Design review of the part shown in the three views and the two pictorial views. Dimensions are in mm from the part's minimum x, y and z. A direction names the side the tool comes from. Coordinates: 2 decimals unless noted, no trailing zeros. Write each loop counter-clockwise with the first axis right and the second up, starting at its lowest first coordinate (ties: lowest second). Pieces come first, ordered by that corner, then holes.
Q1. For pin 1 Ø5 at (x, y) = (6.5, 16.5) entering from +Z; pin 2 Ø2 at (x, y) = (15, 5) entering from +Z; pin 3 Ø1.8 at (x, y) = (9.5, 9) entering from +Z; pin 4 Ø2 at (x, z) = (4, 2) entering from -Y, all flat-tipped, find the tip position at first contact; note any pin that passes through.
Q2. For L1, parallel to X at y = 5, z = 0.9; L2, parallel to Y at x = 5.75, z = 0.2; L3, parallel to Y at x = 10, z = 3.2, list the stretches that pass through material, from the lowest coordinate up.
Q3. Take a section at A-A, the plane x = 10. Write out the cut boundary in (y, z), plus the area to 3 significant figures.
Q4. Take a section at D-D, the plane x = 5.25. Write out the cut boundary in (y, z), plus the area to 3 significant figures.
Q5. The part is to be moulded in two halves that separate along Y. For the marked faces 1, 2 and 3, say which applies: released by +Y, released by -Y, zero draft, split by the parting line, or undercut.
Q6. Take a section at C-C, the plane z = 0.65. Write out the cut boundary in (x, y), plus the area to 3 significant figures.
Q7. For the marked faces 4 and 5, list the 3-axis set-ups (+Z, -Z, +X, -X, +Y, -Y) from which the entire face can be reached by the end or side of a thin tool; tool diameter is ignored.
Q8. Take a section at B-B, the plane y = 9. Write out the cut boundary in (x, z), plus the area to 3 significant figures.
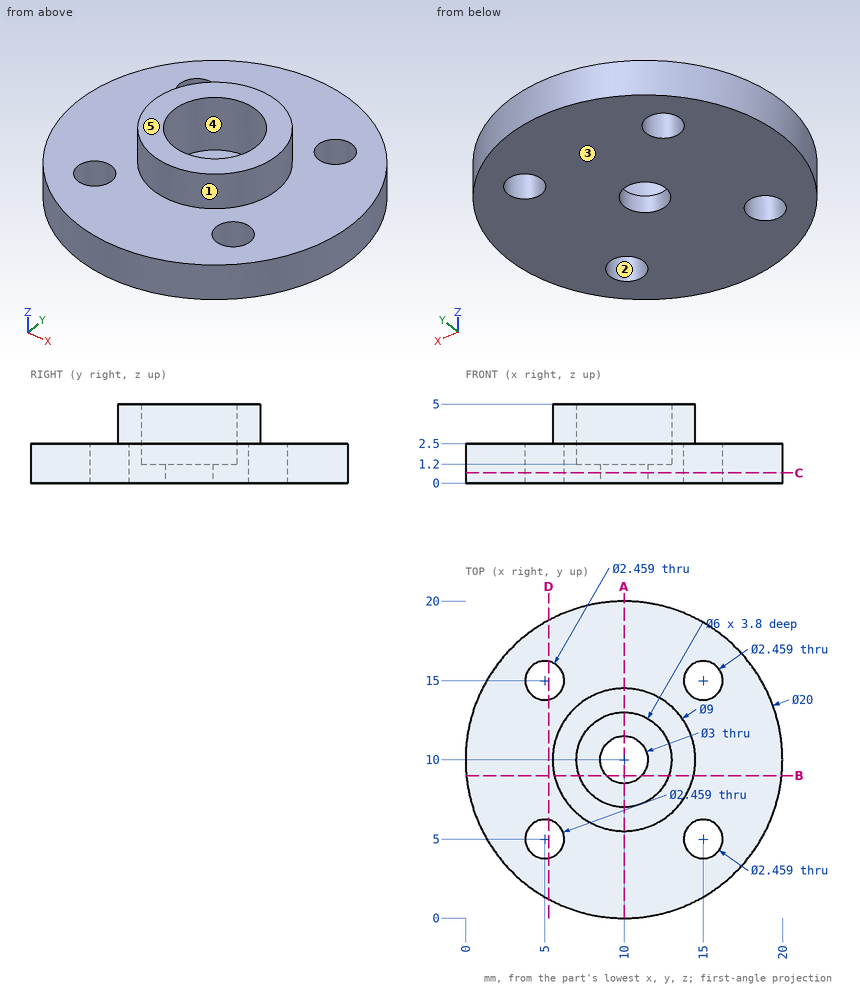
Responses:
1. pin 1: stops at z = 2.5
1. pin 2: passes through
1. pin 3: stops at z = 1.2
1. pin 4: stops at y = 1.34
2. L1: x = 1.34 to 3.77, 6.23 to 13.77, 16.23 to 18.66
2. L2: y = 0.95 to 4.03, 5.97 to 14.03, 15.97 to 19.05
2. L3: y = 5.5 to 7, 13 to 14.5
3. outline: (0, 0) - (8.5, 0) - (8.5, 1.2) - (7, 1.2) - (7, 5) - (5.5, 5) - (5.5, 2.5) - (0, 2.5) - close; (11.5, 0) - (20, 0) - (20, 2.5) - (14.5, 2.5) - (14.5, 5) - (13, 5) - (13, 1.2) - (11.5, 1.2) - close
3. area: 46.1 mm2
4. outline: (1.2, 0) - (3.8, 0) - (3.8, 2.5) - (1.2, 2.5) - close; (6.2, 0) - (13.8, 0) - (13.8, 2.5) - (6.2, 2.5) - close; (16.2, 0) - (18.8, 0) - (18.8, 2.5) - (16.2, 2.5) - close
4. area: 32.0 mm2
5. face 1: split by the parting line
5. face 2: undercut
5. face 3: zero draft
6. outline: circle Ø20 at (10, 10); hole circle Ø2.46 at (5, 5); hole circle Ø2.46 at (5, 15); hole circle Ø3 at (10, 10); hole circle Ø2.46 at (15, 5); hole circle Ø2.46 at (15, 15)
6. area: 288 mm2
7. face 4: +Z
7. face 5: +Z, +X, -X, +Y, -Y
8. outline: (0.05, 0) - (8.88, 0) - (8.88, 1.2) - (7.17, 1.2) - (7.17, 5) - (5.61, 5) - (5.61, 2.5) - (0.05, 2.5) - close; (11.12, 0) - (19.95, 0) - (19.95, 2.5) - (14.39, 2.5) - (14.39, 5) - (12.83, 5) - (12.83, 1.2) - (11.12, 1.2) - close
8. area: 47.5 mm2
